from build123d import *

# Parameters (mm, degrees)
SKETCH1_R           = 6.35
BOSS_EXTRUDE1_DEPTH = 421.64
SKETCH2_R           = 10.795
BOSS_EXTRUDE2_DEPTH = 421.64
SKETCH3_R           = 25.4
SKETCH3_R_2         = 6.35
CUT_EXTRUDE1_DEPTH  = 52.324
CUT_EXTRUDE2_START  = -57.658
SKETCH4_R           = 25.4
SKETCH4_R_2         = 6.35
CUT_EXTRUDE2_DEPTH  = 57.658
CHAMFER1_SIZE       = 6.35


with BuildPart() as part:
    # Sketch1 → Boss-Extrude1 (new body)
    with BuildSketch(Plane(origin=(0, 0, 0), x_dir=(1, 0, 0), z_dir=(0, 1, 0))):
        with Locations(Location((0, 0, 0), (0, 0, 270))):
            Circle(SKETCH1_R)
    extrude(amount=BOSS_EXTRUDE1_DEPTH)

    # Sketch2 → Boss-Extrude2 (add)
    with BuildSketch(Plane(origin=(0, 0, 0), x_dir=(-1, 0, 0), z_dir=(0, -1, 0))):
        with Locations(Location((0, 0, 0), (0, 0, 90))):
            Circle(SKETCH2_R)
    extrude(amount=-BOSS_EXTRUDE2_DEPTH)

    # Sketch3 → Cut-Extrude1 (cut)
    with BuildSketch(Plane.XZ):
        Circle(SKETCH3_R)
        with Locations(Location((0, 0, 0), (0, 0, 270))):
            Circle(SKETCH3_R_2, mode=Mode.SUBTRACT)
    extrude(amount=-CUT_EXTRUDE1_DEPTH, mode=Mode.SUBTRACT)

    # Sketch4 → Cut-Extrude2 (cut)
    with BuildSketch(Plane(origin=(0, 421.64, 0), x_dir=(1, 0, 0), z_dir=(0, 1, 0)).offset(CUT_EXTRUDE2_START)):
        Circle(SKETCH4_R)
        with Locations(Location((0, 0, 0), (0, 0, 90))):
            Circle(SKETCH4_R_2, mode=Mode.SUBTRACT)
    extrude(amount=CUT_EXTRUDE2_DEPTH, mode=Mode.SUBTRACT)

    # Chamfer1
    # the kernel refuses this chamfer: 6.35 mm, written as the material it takes off along each edge
    with BuildSketch(Plane(origin=(0, 52.324, 0), x_dir=(0, 0, -1), z_dir=(-1, 0, 0))) as chamfer1_piece_1_section:
        Polygon((10.795, -CHAMFER1_SIZE), (10.795 - CHAMFER1_SIZE, 0), (10.795, 0), align=None)
    chamfer1_piece_1 = revolve(axis=Axis((0, 52.324, 0), (0, -1, 0)), mode=Mode.PRIVATE)
    chamfer1_piece_1 = chamfer1_piece_1 - Plane(origin=(0, 56.4676015, 0), x_dir=(0, 0, -1), z_dir=(0, -1, 0)) * Cylinder(6.35, 44, mode=Mode.PRIVATE)
    add(chamfer1_piece_1, mode=Mode.SUBTRACT)
    with BuildSketch(Plane(origin=(0, 363.982, 0), x_dir=(0, 0, -1), z_dir=(-1, 0, 0))) as chamfer1_piece_2_section:
        Polygon((10.795, CHAMFER1_SIZE), (10.795 - CHAMFER1_SIZE, 0), (10.795, 0), align=None)
    chamfer1_piece_2 = revolve(axis=Axis((0, 363.982, 0), (0, -1, 0)), mode=Mode.PRIVATE)
    chamfer1_piece_2 = chamfer1_piece_2 - Plane(origin=(0, 359.8383985, 0), x_dir=(0, 0, -1), z_dir=(0, -1, 0)) * Cylinder(6.35, 44, mode=Mode.PRIVATE)
    add(chamfer1_piece_2, mode=Mode.SUBTRACT)


solid = part.part
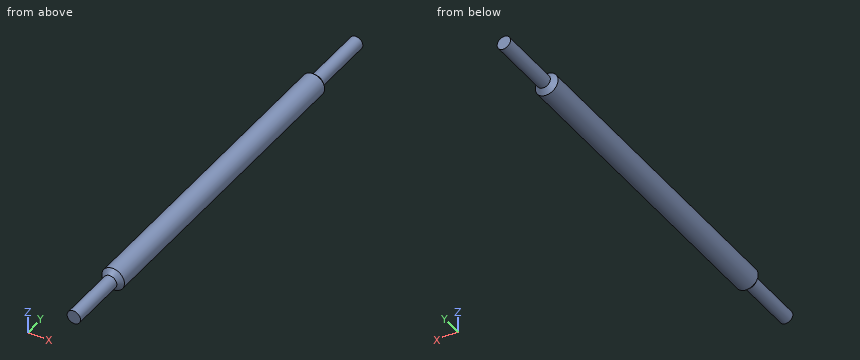
Read the model definition and answer for the solid it produces. Units are mm, in the model's axes. Round coordinates to 2 decimals unless told otherwise and drop trailing zeros. Write each loop counter-clockwise with the first axis right and the second up, starting at its lowest first coordinate (ties: lowest second). Pieces come first, ordered by that corner, then holes.
1. The part is cut by section A-A, the plane x = 0. Determine the outline of the cut face in (y, z) (3 decimals).
2. Straight lines are drawn through the part: L1, parallel to X at y = 293, z = -1.25; L2, parallel to X at y = 289.5, z = 0 (3 decimals); L3, parallel to Z at x = -0.5, y = 33. For each, find the intervals that lie inside material, in ascending order.
3. The part is cut by section D-D, the plane y = 151.5. Determine the outline of the cut face in (x, z) (3 decimals), then the cut area to 3 significant figures.
4. The part is cut by section C-C, the plane y = 392.5. Determine the outline of the cut face in (x, z).
5. The part is cut by section B-B, the plane z = 0. Determine the outline of the cut face in (x, y) (3 decimals).
6. Given pin 1 Ø1 at (y, z) = (257.5, -5) entering from -X; pin 2 Ø4 at (x, y) = (4.5, 324.5) entering from +Z; pin 3 Ø12 at (x, y) = (-7, 45) entering from -Z, each flat-ended and moving along its own axis, determine where each tip first touches the part or whether it passes through.
Values:
1. outline: (0, -6.35) - (54.229, -6.35) - (58.674, -10.795) - (357.632, -10.795) - (362.077, -6.35) - (421.64, -6.35) - (421.64, 6.35) - (362.077, 6.35) - (357.632, 10.795) - (58.674, 10.795) - (54.229, 6.35) - (0, 6.35) - close
2. L1: x = -10.72 to 10.72
2. L2: x = -10.795 to 10.795
2. L3: z = -6.33 to 6.33
3. outline: circle Ø21.59 at (0, 0)
3. area: 366 mm2
4. outline: circle Ø12.7 at (0, 0)
5. outline: (-10.795, 58.674) - (-6.35, 54.229) - (-6.35, 0) - (6.35, 0) - (6.35, 54.229) - (10.795, 58.674) - (10.795, 357.632) - (6.35, 362.077) - (6.35, 421.64) - (-6.35, 421.64) - (-6.35, 362.077) - (-10.795, 357.632) - close
6. pin 1: stops at x = -9.81
6. pin 2: stops at z = 10.5
6. pin 3: stops at z = -6.27
